Verification items for the finished model (mm, model axes). Give positions to 0.01 mm unless a question says otherwise; leave off trailing zeros. Loops run counter-clockwise (first coordinate to the right, second up) from the corner with the lowest first, then second, coordinate; pieces in that order, holes last. Notation, with made-up numbers: M 50.5,-2.5 L 56.5,-2.5 A18 cw 56.5,6.5 Z; hole C 19.5,49 d3. An arc over 180 degrees is marked long. Answer in a Markdown table with one row per item.
Autodesk Inventor part; units mm, degrees
ref_plane "YZ Plane" through (0, 0, 0) normal (1, 0, 0) x (0, 1, 0)
ref_plane "XZ Plane" through (0, 0, 0) normal (0, 1, 0) x (-1, 0, 0)
ref_plane "XY Plane" through (0, 0, 0) normal (0, 0, 1) x (1, 0, 0)
sketch "Sketch1" plane through (0, 0, 0) normal (0, 1, 0) x (-1, 0, 0)
  circle A0 centre (0, 0) radius 114.3
  circle A1 centre (0, 0) radius 107.95
  line L0 (-63.5, -63.5) -> (63.5, -63.5)
  line L1 (63.5, -63.5) -> (63.5, 63.5)
  line L2 (63.5, 63.5) -> (-63.5, 63.5)
  line L3 (-63.5, 63.5) -> (-63.5, -63.5)
  line L4 (-63.5, -63.5) -> (63.5, 63.5) construction
  line L5 (63.5, -63.5) -> (-63.5, 63.5) construction
  line L6 (57.15, 57.15) -> (57.15, -57.15)
  line L7 (57.15, -57.15) -> (-57.15, -57.15)
  line L8 (-57.15, -57.15) -> (-57.15, 57.15)
  line L9 (-57.15, 57.15) -> (57.15, 57.15)
  dimension "d0" = 228.6
  dimension "d1" = 6.35
  dimension "d2" = 127
  dimension "d3" = 127
  dimension "d4" = 6.35
extrude "Extrusion1" add sketch "Sketch1" along normal blind 6.35 contours A1
extrude "Extrusion2" add sketch "Sketch1" along normal blind 12.7 contours A0
extrude "Extrusion3" add sketch "Sketch1" along normal blind 6.35 contours L3 L2 L1 L0 | L6 L7 L8 L9
properties part number "Drainage Base"
Item 1: Go/stop test with flat-tipped pins: pin 1 (3 mm diameter, centred on y = 10, z = 32, fed in from -X); pin 2 (5 mm diameter, centred on x = 15.5, z = -63.5, fed in from +Y); pin 3 (6 mm diameter, centred on x = 8, y = 9.5, fed in from +Z). Record where each tip stops, or that it passes through.
Reported:
| item | result |
|---|---|
| pin 1 | stops at x = -110.16 |
| pin 2 | stops at y = 6.35 |
| pin 3 | stops at z = 114.19 |
Item 2: Scan lines: L1, parallel to Z at x = 0, y = 11.75; L2, parallel to Y at x = 23, z = 58; L3, parallel to X at y = 7.75, z = 45. Record each from-to range of solid material in increasing order. Write a range as [from, to].
Reported:
| item | result |
|---|---|
| L1 | z = [-114.3, -107.95], [107.95, 114.3] |
| L2 | y = [0, 6.35] |
| L3 | x = [-105.07, -98.12], [98.12, 105.07] |
Item 3: Release check for a two-part mould opening along Z. For faces 1 (the flat face through (2, 6.35, 2)), 2 (the cylindrical face through (79.56, 9.48, -72.96)), 3 (the cylindrical face through (114.19, 6.26, -5.03)), 4 (the flat face through (-84.1, 12.7, 68.3)) record: released by +Z, released by -Z, zero draft, split by the parting line, or undercut.
Reported:
| item | result |
|---|---|
| face 1 | undercut |
| face 2 | undercut |
| face 3 | split by the parting line |
| face 4 | zero draft |
Item 4: Sectioned sample at B-B (z = 0). Record the cut outline in (x, y), and give its area (3 significant figures).
Reported:
| item | result |
|---|---|
| outline | M -114.3,0 L 114.3,0 L 114.3,12.7 L 107.95,12.7 L 107.95,6.35 L -107.95,6.35 L -107.95,12.7 L -114.3,12.7 Z |
| area | 1,530 mm^2 |
Item 5: Sectioned sample at C-C (y = 10). Record the cut outline in (x, z), and give its area (3 significant figures).
Reported:
| item | result |
|---|---|
| outline | C 0,0 d228.6; hole C 0,0 d215.9 |
| area | 4,430 mm^2 |
Item 6: Sectioned sample at A-A (x = 0). Record the cut outline in (y, z).
Reported:
| item | result |
|---|---|
| outline | M 0,-114.3 L 12.7,-114.3 L 12.7,-107.95 L 6.35,-107.95 L 6.35,107.95 L 12.7,107.95 L 12.7,114.3 L 0,114.3 Z |
